Build history of the part. All positions in model axes, mm. Face numbers are marked on the shaded views. A direction names the side the tool comes from. Coordinates: 2 decimals unless noted, no trailing zeros. Order: outer loops, then holes, each group sorted by start corner. A loop starts at its lowest first (then second) coordinate and runs counter-clockwise, first axis right, second up. Notation, with made-up numbers: (10, -39) - (42, -39) arc R33 cw to (42, -7) - close; hole circle Ø4 at (67.25, -28). An arc over 180 degrees is marked (long way). Return JSON: item names as keys, results as strings.
Autodesk Fusion 360 part; units mm, degrees
sketch "Sketch1" plane through (0, 0, 0) normal (0, 0, 1) x (1, 0, 0)
  line L0 (0, 3) -> (10, 3)
  line L1 (10, 3) -> (10, 0)
  line L2 (10, 0) -> (14, 0)
  line L3 (14, 0) -> (14, 4.5)
  line L4 (14, 4.5) -> (15, 4.5)
  line L5 (15, 4.5) -> (15, 29)
  line L6 (15, 29) -> (0, 29)
  line L7 (0, 29) -> (0, 3)
  dimension "d1" = 30
  dimension "d2" = 29
  dimension "d3" = 28
  dimension "d4" = 20
  dimension "d5" = 3
  dimension "d6" = 4.5
revolve "Revolve1" add sketch "Sketch1" angle 360 about axis through (0, 29, 0) along (0, -1, 0)
chamfer "Chamfer1" distance 1 angle 45 2 edges at (-13.9849, 4.5, -5.4242) (-13.0526, 0, -5.0626)
sketch "Sketch2" plane through (0, 3, 0) normal (0, -1, 0) x (1, 0, 0)
  circle A0 centre (0, 0) radius 10
hole "Hole1" at (0, 3, 0) direction (0, 1, 0) diameter 6 depth 14 tip angle 118
sketch "Sketch3" plane through (0, 0, 0) normal (0, 0, 1) x (1, 0, 0)
  line L0 (13, 0) -> (-13, 0)
  point P0 (0, 9.3)
  dimension "d12" = 9.3
hole "Hole2" at (0, 9.3, 0) direction (0, 0, -1) diameter 2.529 end through all
chamfer "Chamfer2" distance 0.3 angle 45 1 edges at (1.0848, 3, 2.797)
fillet "Fillet1" radius 1 1 edges at (-13.9849, 29, -5.4242)
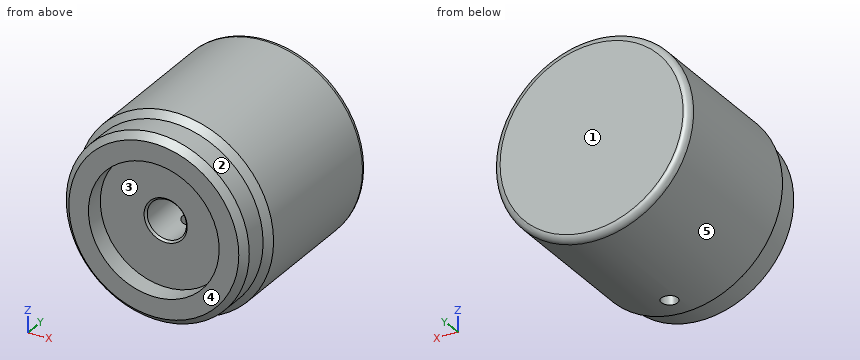
1. Mould opens along Z. For the marked faces 3, 4 and 5 say: pulls with the +Z half, pulls with the -Z half, needs draft (parallel to the pull), parting line crosses it, or undercut.
Check values:
{"face 3": "undercut", "face 4": "needs draft", "face 5": "parting line crosses it"}
2. Probe L1, parallel to Y at x = 0, z = -9.75; L2, parallel to Z at x = -7.5, y = 9.5; L3, parallel to Z at x = 0, y = 6. List the from-to ranges inside material, lowest first.
Check values:
{"L1": "3 to 8.04, 10.56 to 29", "L2": "-12.99 to 12.99", "L3": "-15 to -3, 3 to 15"}
3. Drop flat-ended pins along their axis: pin 1 (3 mm diameter, centred on y = 14, z = -9, fed in from -X); pin 2 (3.5 mm diameter, centred on x = 0, z = 0, fed in from -Y); pin 3 (12 mm diameter, centred on y = 5.5, z = -1.5, fed in from +X); pin 4 (5 mm diameter, centred on y = 23.5, z = 7, fed in from -X). Give the stop position or say it passes through.
Check values:
{"pin 1": "x = -12.99", "pin 2": "y = 17.75", "pin 3": "x = 15", "pin 4": "x = -14.31"}
4. Tool access for the marked faces 1 and 2: list every direction of +Z, -Z, +X, -X, +Y, -Y with a clear straight run to the whole face (end or side of a thin tool).
Check values:
{"face 1": "+Z, -Z, +X, -X, +Y", "face 2": "-Y"}
5. Cut at A-A on y = 13. Give the cut face in (x, z).
Check values:
{"outline": "circle Ø30 at (0, 0); hole circle Ø6 at (0, 0)"}
6. Cut at B-B on y = 8.5. Give the cut face in (x, z), plus the area to 3 significant figures.
Check values:
{"outline": "(-0.98, -14.97) - (-0.98, -2.84) arc R3 cw (long way) to (0.98, -2.84) - (0.98, -14.97) arc R15 ccw (long way) to start", "area": "655 mm²"}
7. Cut at C-C on y = 17.75. Give the cut face in (x, z).
Check values:
{"outline": "circle Ø30 at (0, 0); hole circle Ø3.5 at (0, 0)"}
